Study the drawing (mm; zero at the part's minimum x, y, z) and answer. A direction names the side the tool comes from. Give positions to 0.01 mm unless a question says otherwise; leave off trailing zeros. Order: outer loops, then holes, each group sorted by start corner. A loop starts at its lowest first (then second) coordinate and runs counter-clockwise, first axis right, second up.
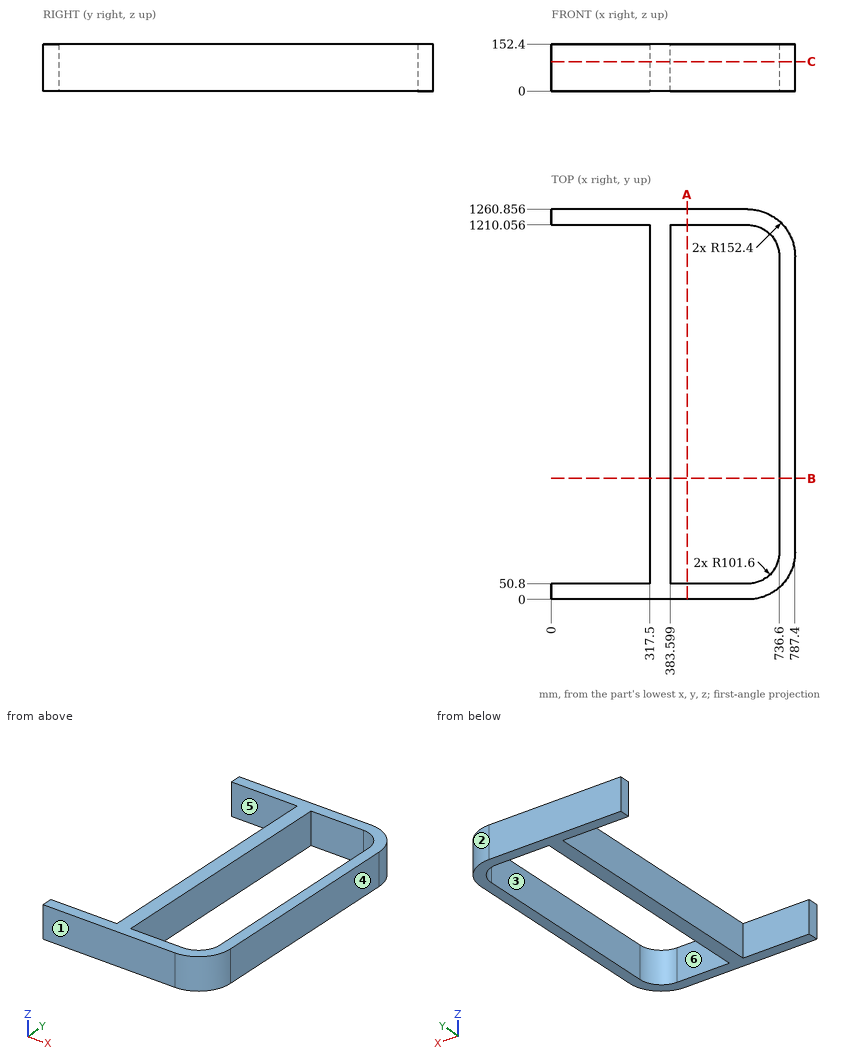
1) Find section B-B (y = 391). Write down the section's boundary in (x, z), then the cut area to 3 significant figures.
Geometry says:
outline: (317.5, 0) - (383.6, 0) - (383.6, 152.4) - (317.5, 152.4) - close; (736.6, 0) - (787.4, 0) - (787.4, 152.4) - (736.6, 152.4) - close
area: 17,800 mm2
2) A tool of negligible diameter and unlimited length cuts with its end or side. For the marked faces 4, 5 and 6, from which of +Z, -Z, +X, -X, +Y, -Y can it reach the whole face along a straight path? Write none if from no direction.
Geometry says:
face 4: +Z, -Z, +X, +Y, -Y
face 5: +Z, -Z, -X
face 6: +Z, -Z
3) Straight lines are drawn through the part: probe 1 along X at (y, z) = (445.5, 140); probe 2 along Y at (x, z) = (315.5, 88); probe 3 along X at (y, z) = (101, 39.5). For each, find the intervals that lie inside material, in ascending order.
Geometry says:
probe 1: x = 317.5 to 383.6, 736.6 to 787.4
probe 2: y = 0 to 50.8, 1210.06 to 1260.86
probe 3: x = 317.5 to 383.6, 722.64 to 778.47
4) For a pull along Y with two mould halves and no side action, classify the marked faces 1, 2 and 3 as +Y half, -Y half, draft (parallel to the pull), parting line (faces both ways), or undercut.
Geometry says:
face 1: -Y half
face 2: +Y half
face 3: undercut
5) Given P1, Ø8, axis at y = 524.5, z = 68.5, coming from the -X side; P2, Ø1, axis at x = 656, z = 88, coming from the +Y side, each flat-ended and moving along its own axis, determine where each tip first touches the part or whether it passes through.
Geometry says:
P1: stops at x = 317.5
P2: stops at y = 1259.47
6) Find section C-C (z = 95.5). Write down the section's boundary in (x, y), then the cut area to 3 significant figures.
Geometry says:
outline: (0, 0) - (635, 0) arc R152.4 ccw to (787.4, 152.4) - (787.4, 1108.46) arc R152.4 ccw to (635, 1260.86) - (0, 1260.86) - (0, 1210.06) - (317.5, 1210.06) - (317.5, 50.8) - (0, 50.8) - close; hole (383.6, 50.8) - (635, 50.8) arc R101.6 ccw to (736.6, 152.4) - (736.6, 1108.46) arc R101.6 ccw to (635, 1210.06) - (383.6, 1210.06) - close
area: 210,000 mm2
7) Find section A-A (x = 439). Write down the section's boundary in (y, z).
Geometry says:
outline: (0, 0) - (50.8, 0) - (50.8, 152.4) - (0, 152.4) - close; (1210.06, 0) - (1260.86, 0) - (1260.86, 152.4) - (1210.06, 152.4) - close
